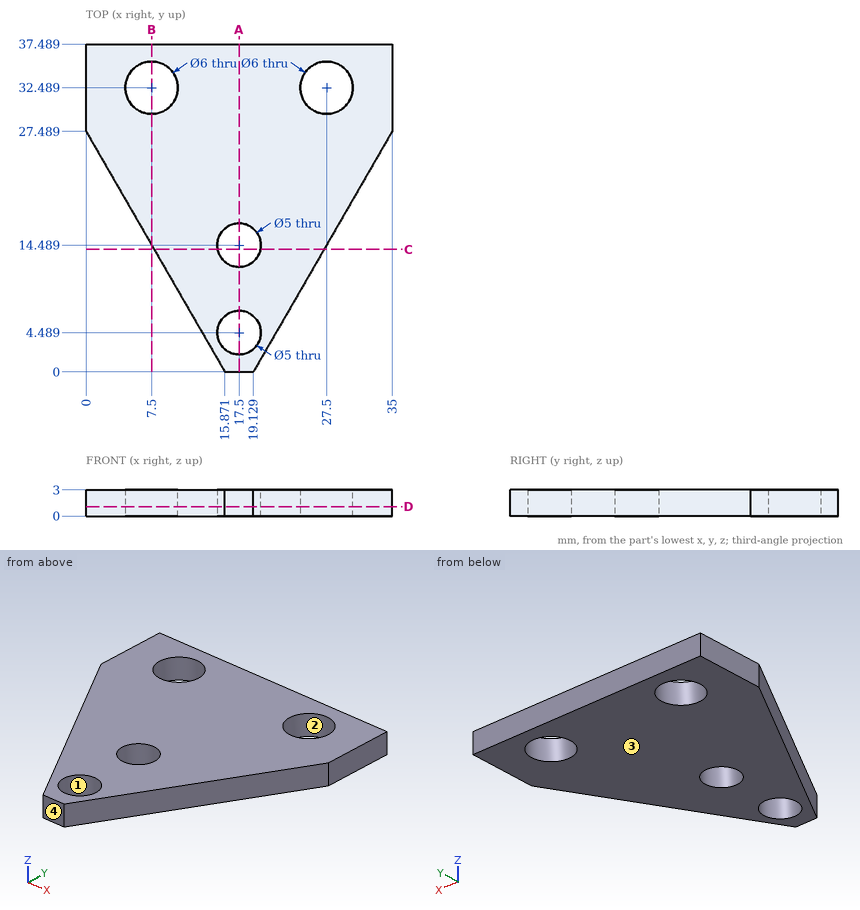
Study the drawing (mm; zero at the part's minimum x, y, z) and answer. Give positions to 0.01 mm unless a question says otherwise; leave off trailing zeros. Order: outer loops, then holes, each group sorted by start corner. A loop starts at its lowest first (then second) coordinate and runs counter-clockwise, first axis right, second up. Notation, with made-up numbers: M 32.25,75 L 51.25,75 A18 cw 51.25,102 Z; hole C -9.5,28.25 d10. An arc over 180 degrees is marked long. Put each result on its own line as item: value. Start each with the question number.
Item 1: The part is cut by section B-B, the plane x = 7.5. Determine the outline of the cut face in (y, z), and give its area (3 significant figures).
Item 2: A flat-ended cylindrical pin translates along its axis: P1, Ø4.5, axis at x = 17.5, y = 14.49, coming from the -Z side. Find the tip coordinate at first contact, or state that the pin passes through.
Item 3: The part is cut by section D-D, the plane z = 1.1. Determine the outline of the cut face in (x, y).
Item 4: Find the intervals of material crossed by line 1 along Y through (x, z) = (17.5, 2.4); line 2 along X through (y, z) = (32, 2.4); line 3 along Y through (x, z) = (18, 1.45), in increasing order.
Item 5: The part is cut by section A-A, the plane x = 17.5. Determine the outline of the cut face in (y, z).
Item 6: For a pull along Y with two mould halves and no side action, classify the marked faces 1, 2, 3 and 4 as +Y half, -Y half, draft (parallel to the pull), parting line (faces both ways), or undercut.
Item 7: The part is cut by section C-C, the plane y = 14. Determine the outline of the cut face in (x, z).
Answer key:
1. outline: M 14.5,0 L 29.49,0 L 29.49,3 L 14.5,3 Z; M 35.49,0 L 37.49,0 L 37.49,3 L 35.49,3 Z
1. area: 51.0 mm²
2. P1: passes through
3. outline: M 0,27.49 L 15.87,0 L 19.13,0 L 35,27.49 L 35,37.49 L 0,37.49 Z; hole C 7.5,32.49 d6; hole C 17.5,4.49 d5; hole C 17.5,14.49 d5; hole C 27.5,32.49 d6
4. line 1: y = 0 to 1.99, 6.99 to 11.99, 16.99 to 37.49
4. line 2: x = 0 to 4.54, 10.46 to 24.54, 30.46 to 35
4. line 3: y = 0 to 2.04, 6.94 to 12.04, 16.94 to 37.49
5. outline: M 0,0 L 1.99,0 L 1.99,3 L 0,3 Z; M 6.99,0 L 11.99,0 L 11.99,3 L 6.99,3 Z; M 16.99,0 L 37.49,0 L 37.49,3 L 16.99,3 Z
6. face 1: undercut
6. face 2: undercut
6. face 3: draft
6. face 4: -Y half
7. outline: M 7.79,0 L 15.05,0 L 15.05,3 L 7.79,3 Z; M 19.95,0 L 27.21,0 L 27.21,3 L 19.95,3 Z
